Here's how the part is built. I have some questions about the finished solid (model axes, mm). Face numbers are marked on the shaded views. A direction names the side the tool comes from. Round coordinates to 2 decimals unless told otherwise and drop trailing zeros. Order: outer loops, then holes, each group sorted by start corner. A loop starts at its lowest first (then second) coordinate and runs counter-clockwise, first axis right, second up. Notation, with made-up numbers: (34.5, 69.5) - (53.5, 69.5) arc R8 ccw to (53.5, 77.5) - close; hole circle Ø7 at (-13.75, -38). An arc over 180 degrees is marked (long way). One line per item, written item: value.
Autodesk Inventor part; units mm, degrees
ref_plane "YZ Plane" through (0, 0, 0) normal (1, 0, 0) x (0, 1, 0)
ref_plane "XZ Plane" through (0, 0, 0) normal (0, 1, 0) x (-1, 0, 0)
ref_plane "XY Plane" through (0, 0, 0) normal (0, 0, 1) x (1, 0, 0)
sketch "스케치5" plane through (0, 0, 0) normal (1, 0, 0) x (0, 1, 0)
  circle A0 centre (0, 0) radius 10
  dimension "d11" = 20
extrude "돌출4" add sketch "스케치5" along normal mid plane 50
sketch "스케치6" plane through (0, 0, 0) normal (0, 1, 0) x (-1, 0, 0)
  line L0 (25, 10) -> (-25, 10)
  line L1 (25, -10) -> (-25, -10)
  line L2 (-10, 10) -> (10, 10)
  line L3 (10, 10) -> (10, -10)
  line L4 (10, -10) -> (-10, -10)
  line L5 (-10, -10) -> (-10, 10)
  line L6 (25, -10) -> (25, 10)
  point P0 (0, 0)
  dimension "d14" = 20
  dimension "d15" = 15
extrude "돌출5" add sketch "스케치6" along normal blind 70 contours L3 L1 L5 L0
sketch "스케치7" plane through (0, 70, 0) normal (0, 1, 0) x (1, 0, 0)
  circle A0 centre (0, 0) radius 10
  dimension "d18" = 20
extrude "돌출6" add sketch "스케치7" along normal blind 10
sketch "스케치8" plane through (0, 80, 0) normal (0, 1, 0) x (1, 0, 0)
  circle A0 centre (0, 0) radius 10
  line L0 (10, -10) -> (10, 0)
  line L1 (-10, 0) -> (10, 0)
revolve "회전2" add sketch "스케치8" angle 360 about axis through (-10, 80, 0) along (1, 0, 0) picked at (2.495, 2.2104) contours L1 A0
properties part number "L3_0.1" material "ABS 플라스틱"
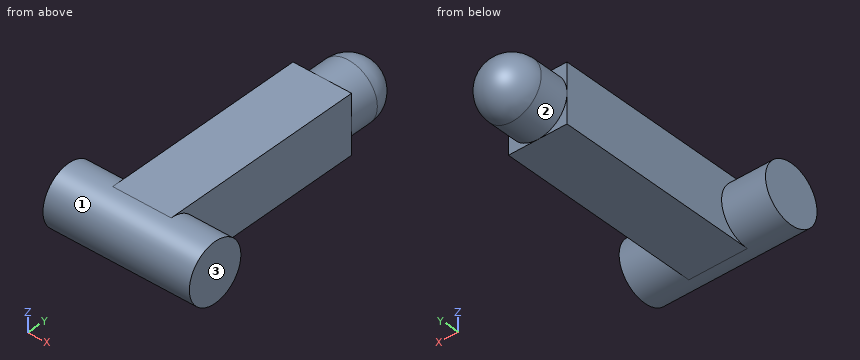
Q1. If we section it at D-D, the plane x = 3.5: Please give me the cut outline in (y, z) (1 decimal).
Results list:
outline: (0, -10) - (70, -10) - (70, -9.4) - (80, -9.4) arc R9.4 ccw to (80, 9.4) - (70, 9.4) - (70, 10) - (0, 10) arc R10 ccw to start
Q2. Will these pins go through, and if not, where does the flat tip stop? pin 1 (5 mm diameter, centred on x = 3, z = 7, fed in from +Y); pin 2 (12 mm diameter, centred on y = 25, z = 1.5, fed in from -X); pin 3 (1.5 mm diameter, centred on x = -10.5, y = 4, fed in from -Z); pin 4 (5 mm diameter, centred on x = 5, z = -4.5, fed in from +Y).
Results list:
pin 1: y = 88.59
pin 2: x = -10
pin 3: z = -10
pin 4: y = 89.06
Q3. If we section it at B-B, the plane y = 71.5: Please give me the cut outline in (x, z), then the cut area to 3 significant figures.
Results list:
outline: circle Ø20 at (0, 0)
area: 314 mm²
Q4. If we section it at A-A, the plane x = -6: Please give me the cut outline in (y, z).
Results list:
outline: (0, -10) - (70, -10) - (70, -8) - (80, -8) arc R8 ccw to (80, 8) - (70, 8) - (70, 10) - (0, 10) arc R10 ccw to start
Q5. If I drill on line 1 along X through (y, z) = (67.5, -7.25); line 2 along X through (y, z) = (71, 7.25); line 3 along Z through (x, y) = (21.5, -5), over which ranges is the centre line in solid material (lowest first)?
Results list:
line 1: -10 to 10
line 2: -6.89 to 6.89
line 3: -8.66 to 8.66
Q6. Which directions (+Z, -Z, +X, -X, +Y, -Y) give clear straight access to the entire face, cutting with the end or side of a thin tool? Please do the marked faces 1, 2 and 3.
Results list:
face 1: none
face 2: +Y
face 3: +Z, -Z, +X, +Y, -Y
Q7. If we section it at C-C, the plane z = 3: Please give me the cut outline in (x, y), then the cut area to 3 significant figures.
Results list:
outline: (-25, -9.54) - (25, -9.54) - (25, 9.54) - (10, 9.54) - (10, 70) - (9.54, 70) - (9.54, 80) arc R9.54 ccw to (-9.54, 80) - (-9.54, 70) - (-10, 70) - (-10, 9.54) - (-25, 9.54) - close
area: 2,500 mm²
